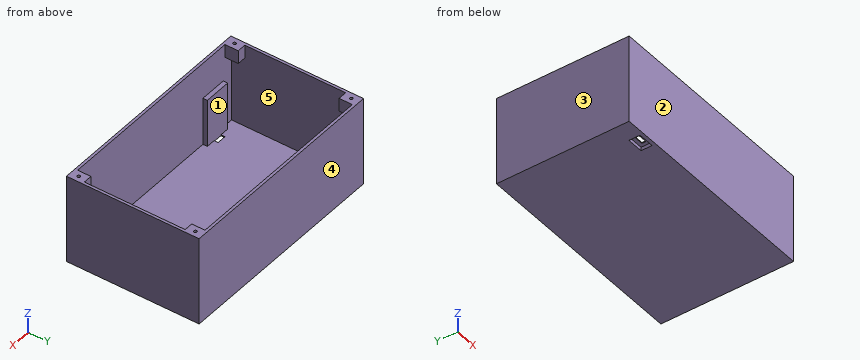
Autodesk Inventor part; units mm, degrees
ref_plane "YZ Plane" through (0, 0, 0) normal (1, 0, 0) x (0, 1, 0)
ref_plane "XZ Plane" through (0, 0, 0) normal (0, 1, 0) x (-1, 0, 0)
ref_plane "XY Plane" through (0, 0, 0) normal (0, 0, 1) x (1, 0, 0)
sketch "Sketch7" plane through (0, 0, 0) normal (0, 0, 1) x (1, 0, 0)
  line L0 (125, -75) -> (-125, -75)
  line L1 (-125, -75) -> (-125, 75)
  line L2 (-125, 75) -> (125, 75)
  line L3 (125, 75) -> (125, -75)
  line L4 (125, -75) -> (-125, 75) construction
  line L5 (-125, -75) -> (125, 75) construction
  point P0 (0, 0)
  dimension "d15" = 250
  dimension "d16" = 150
extrude "Box Outside" add sketch "Sketch7" along normal blind 100
sketch "Sketch8" plane through (0, 0, 100) normal (0, 0, 1) x (1, 0, 0)
  line L0 (-122, 72) -> (122, 72)
  line L1 (122, 72) -> (122, -72)
  line L2 (122, -72) -> (-122, -72)
  line L3 (-122, -72) -> (-122, 72)
  line L4 (125, 75) -> (-125, 75)
  line L5 (-125, 75) -> (-125, -75)
  line L6 (-125, -75) -> (125, -75)
  line L7 (125, -75) -> (125, 75)
  point P0 (0, 0)
  dimension "d19" = 3
  dimension "d20" = 3
  dimension "d21" = 3
  dimension "d22" = 3
extrude "Box Cut" cut sketch "Sketch8" against normal blind 95 contours L0 L1 L2 L3
sketch "Sketch9" plane through (-122, -72, 100) normal (0, 1, 0) x (1, 0, 0)
  line L0 (0, 0) -> (10, 0)
  line L1 (10, 0) -> (10, 15)
  line L2 (10, 15) -> (0, 15)
  line L3 (0, 15) -> (0, 0)
  point P0 (122, 100)
  dimension "d25" = 10
  dimension "d26" = 15
extrude "ScrewHole Box LB" add sketch "Sketch9" along normal blind 15
sketch "Sketch10" plane through (-122, -72, 5) normal (0, 1, 0) x (1, 0, 0)
  line L0 (244, -95) -> (244, 0)
  line L1 (244, -95) -> (234, -95)
  line L2 (234, -95) -> (234, -80)
  line L3 (234, -80) -> (244, -80)
  line L4 (244, -80) -> (244, -95)
  point P0 (122, 5)
  dimension "d29" = 10
  dimension "d30" = 15
extrude "ScrewHole Box RB" add sketch "Sketch10" along normal blind 15
sketch "Sketch11" plane through (-122, 72, 100) normal (0, -1, 0) x (1, 0, 0)
  line L0 (0, 0) -> (244, 0)
  line L1 (0, 0) -> (10, 0)
  line L2 (10, 0) -> (10, -15)
  line L3 (10, -15) -> (0, -15)
  line L4 (0, -15) -> (0, 0)
  point P0 (122, -100)
  dimension "d33" = 10
  dimension "d34" = 15
extrude "ScrewHole Box LU" add sketch "Sketch11" along normal blind 15
sketch "Sketch13" plane through (122, -72, 5) normal (-1, 0, 0) x (0, 0, 1)
  line L0 (95, 144) -> (0, 144)
  line L1 (95, 144) -> (80, 144)
  line L2 (80, 144) -> (80, 129)
  line L3 (80, 129) -> (95, 129)
  line L4 (95, 129) -> (95, 144)
  point P0 (-5, 72)
  dimension "d37" = 15
  dimension "d38" = 15
extrude "ScrewHole Box RU" add sketch "Sketch13" along normal blind 10
sketch "Sketch27" plane through (0, 0, 100) normal (0, 0, 1) x (1, 0, 0)
  line L0 (-112, -72) -> (-112, -57)
  line L1 (-125, 75) -> (-125, -75)
  line L2 (-112, -57) -> (-125, -57)
  line L3 (-125, -57) -> (-125, -75)
  line L4 (-125, -75) -> (-112, -75)
  line L5 (-112, -75) -> (-112, -57)
  line L6 (-112, -57) -> (-125, -75)
  line L7 (-112, -75) -> (-125, -57)
  circle A0 centre (-118.5, -66) radius 2.4
  point P0 (0, 0)
  dimension "d84" = 4.8
extrude "Outside ScrewHole LB" cut sketch "Sketch27" against normal blind 26 contours A0 L7 L6 | L6 L7 A0 | A0 L6 L7 | L7 L6 A0
sketch "Sketch29" plane through (0, 0, 100) normal (0, 0, 1) x (1, 0, 0)
  line L0 (-112, -72) -> (-112, -57)
  line L1 (-125, -75) -> (125, -75)
  line L2 (-112, -57) -> (-125, -57)
  line L3 (-125, -57) -> (-125, -75)
  line L4 (-125, -75) -> (-112, -75)
  line L5 (-112, -75) -> (-112, -57)
  line L6 (-112, -57) -> (-125, -75)
  circle A0 centre (-118.5, -66) radius 2.4
  point P0 (0, 0)
extrude "ScrewRibbon LB" add sketch "Sketch29" against normal blind 2 contours A0 L6 | L6 A0
sketch "Sketch30" plane through (0, 0, 100) normal (0, 0, 1) x (1, 0, 0)
  line L0 (-122, -57) -> (-112, -57)
  line L1 (-125, -75) -> (125, -75)
  line L2 (-112, -57) -> (-125, -57)
  line L3 (-125, -57) -> (-125, -75)
  line L4 (-125, -75) -> (-112, -75)
  line L5 (-112, -75) -> (-112, -57)
  line L6 (-112, -57) -> (-125, -75)
  circle A0 centre (-118.5, -66) radius 1.7
  point P0 (0, 0)
  dimension "d92" = 3.4
extrude "Inside ScrewHole LB" cut sketch "Sketch30" against normal blind 24 contours A0 L6 | L6 A0
sketch "Sketch31" plane through (0, 0, 100) normal (0, 0, 1) x (1, 0, 0)
  line L0 (-125, 75) -> (-125, -75)
  line L1 (-112, 57) -> (-122, 57)
  line L2 (-125, 75) -> (-112, 75)
  line L3 (-112, 75) -> (-112, 57)
  line L4 (-112, 57) -> (-125, 57)
  line L5 (-125, 57) -> (-125, 75)
  line L6 (-125, 75) -> (-112, 57)
  circle A0 centre (-118.5, 66) radius 2.4
  point P0 (0, 0)
  dimension "d95" = 4.8
extrude "Outside ScrewHole LU" cut sketch "Sketch31" against normal blind 24 contours A0 L6 | L6 A0
sketch "Sketch32" plane through (0, 0, 100) normal (0, 0, 1) x (1, 0, 0)
  line L0 (-122, 57) -> (-112, 57)
  line L1 (-125, 75) -> (-125, -75)
  line L2 (-112, 57) -> (-125, 57)
  line L3 (-125, 57) -> (-125, 75)
  line L4 (-125, 75) -> (-112, 75)
  line L5 (-112, 75) -> (-112, 57)
  line L6 (-112, 75) -> (-125, 57)
  circle A0 centre (-118.5, 66) radius 2.4
  point P0 (0, 0)
  dimension "d98" = 4.8
extrude "ScrewRibbon LU" add sketch "Sketch32" against normal blind 2 contours A0 L6 | L6 A0
sketch "Sketch33" plane through (0, 0, 100) normal (0, 0, 1) x (1, 0, 0)
  line L0 (125, 75) -> (-125, 75)
  line L1 (-112, 57) -> (-122, 57)
  line L2 (-125, 75) -> (-112, 75)
  line L3 (-112, 75) -> (-112, 57)
  line L4 (-112, 57) -> (-125, 57)
  line L5 (-125, 57) -> (-125, 75)
  line L6 (-125, 75) -> (-112, 57)
  circle A0 centre (-118.5, 66) radius 1.7
  point P0 (0, 0)
  dimension "d101" = 3.4
extrude "Inside ScrewHole LU" cut sketch "Sketch33" against normal blind 21.75 contours A0 L6 | L6 A0
sketch "Sketch34" plane through (0, 0, 100) normal (0, 0, 1) x (1, 0, 0)
  line L0 (112, 57) -> (112, 72)
  line L1 (125, 75) -> (-125, 75)
  line L2 (112, 57) -> (125, 57)
  line L3 (125, 57) -> (125, 75)
  line L4 (125, 75) -> (112, 75)
  line L5 (112, 75) -> (112, 57)
  line L6 (125, 75) -> (112, 57)
  circle A0 centre (118.5, 66) radius 2.4
  point P0 (0, 0)
  dimension "d104" = 4.8
extrude "Outside ScrewHole RU" cut sketch "Sketch34" against normal blind 21.75 contours A0 L6 | L6 A0
sketch "Sketch35" plane through (0, 0, 100) normal (0, 0, 1) x (1, 0, 0)
  line L0 (125, -75) -> (125, 75)
  line L1 (122, 57) -> (112, 57)
  line L2 (125, 75) -> (112, 75)
  line L3 (112, 75) -> (112, 57)
  line L4 (112, 57) -> (125, 57)
  line L5 (125, 57) -> (125, 75)
  line L6 (125, 75) -> (-125, 75)
  line L7 (125, 75) -> (112, 57)
  circle A0 centre (118.5, 66) radius 2.4
  point P0 (0, 0)
  dimension "d107" = 4.8
extrude "ScrewRibbon RU" add sketch "Sketch35" against normal blind 2 contours A0 L7 | L7 A0
sketch "Sketch36" plane through (0, 0, 100) normal (0, 0, 1) x (1, 0, 0)
  line L0 (122, 57) -> (112, 57)
  line L1 (125, -75) -> (125, 75)
  line L2 (112, 57) -> (125, 57)
  line L3 (125, 57) -> (125, 75)
  line L4 (125, 75) -> (112, 75)
  line L5 (112, 75) -> (112, 57)
  line L6 (112, 57) -> (125, 75)
  circle A0 centre (118.5, 66) radius 2.4
  circle A1 centre (118.5, 66) radius 1.7
  point P0 (0, 0)
  dimension "d110" = 3.4
extrude "Inside ScrewHole RU" cut sketch "Sketch36" against normal blind 20 contours A1 L6 | L6 A1
sketch "Sketch37" plane through (0, 0, 100) normal (0, 0, 1) x (1, 0, 0)
  line L0 (125, -75) -> (125, 75)
  line L1 (112, -72) -> (112, -57)
  line L2 (125, -75) -> (112, -75)
  line L3 (112, -75) -> (112, -57)
  line L4 (112, -57) -> (125, -57)
  line L5 (125, -57) -> (125, -75)
  line L6 (112, -75) -> (125, -57)
  circle A0 centre (118.5, -66) radius 2.4
  point P0 (0, 0)
  dimension "d113" = 4.8
extrude "Outside ScrewHole RB" cut sketch "Sketch37" against normal blind 20 contours A0 L6 | L6 A0
sketch "Sketch38" plane through (0, 0, 100) normal (0, 0, 1) x (1, 0, 0)
  line L0 (122, -57) -> (112, -57)
  line L1 (125, -75) -> (125, 75)
  line L2 (112, -57) -> (125, -57)
  line L3 (125, -57) -> (125, -75)
  line L4 (125, -75) -> (112, -75)
  line L5 (112, -75) -> (112, -57)
  line L6 (125, -57) -> (112, -75)
  circle A0 centre (118.5, -66) radius 2.4
  point P0 (0, 0)
  dimension "d116" = 4.8
extrude "ScrewRibbon RB" add sketch "Sketch38" against normal blind 2 contours A0 L6 | L6 A0
sketch "Sketch39" plane through (0, 0, 100) normal (0, 0, 1) x (1, 0, 0)
  line L0 (112, -72) -> (112, -57)
  line L1 (125, -75) -> (125, 75)
  line L2 (112, -57) -> (125, -57)
  line L3 (125, -57) -> (125, -75)
  line L4 (125, -75) -> (112, -75)
  line L5 (112, -75) -> (112, -57)
  line L6 (112, -75) -> (125, -57)
  circle A0 centre (118.5, -66) radius 2.4
  circle A1 centre (118.5, -66) radius 1.7
  point P0 (0, 0)
  dimension "d119" = 3.4
extrude "Inside ScrewHole RB" cut sketch "Sketch39" against normal blind 20 contours A1 L6 | L6 A1
sketch "Sketch42" plane through (-122, -72, 5) normal (0, 1, 0) x (1, 0, 0)
  line L0 (244, 0) -> (0, 0)
  line L1 (12.5963, 0) -> (43.5963, 0)
  line L2 (43.5963, 0) -> (43.5963, -54)
  line L3 (43.5963, -54) -> (12.5963, -54)
  line L4 (12.5963, -54) -> (12.5963, 0)
  point P0 (122, 5)
  point P1 (43.5963, 0)
  dimension "d134" = 31
  dimension "d135" = 54
extrude "ESPHolder" add sketch "Sketch42" along normal blind 5
sketch "Sketch43" plane through (0, 0, 5) normal (0, 0, 1) x (1, 0, 0)
  line L0 (-109.4037, -67) -> (-78.4037, -67)
  line L1 (-99.1037, -67) -> (-88.7037, -67)
  line L2 (-88.7037, -67) -> (-88.7037, -62.5)
  line L3 (-88.7037, -62.5) -> (-99.1037, -62.5)
  line L4 (-99.1037, -62.5) -> (-99.1037, -67)
  line L5 (-78.4037, -67) -> (-109.4037, -67)
  line L6 (-109.4037, -67) -> (-109.4037, -51.7804)
  line L7 (-109.4037, -51.7804) -> (-78.4037, -51.7804)
  line L8 (-78.4037, -51.7804) -> (-78.4037, -67)
  point P0 (0, 0)
  dimension "d138" = 10.3
  dimension "d139" = 10.3
  dimension "d140" = 4.5
extrude "PortHole" cut sketch "Sketch43" against normal through all contours L4 L3 L2 L0
sketch "Sketch44" plane through (0, 0, 0) normal (0, 0, -1) x (-1, 0, 0)
  line L0 (84.7037, -58.5) -> (103.1037, -58.5)
  line L1 (103.1037, -58.5) -> (103.1037, -71)
  line L2 (103.1037, -71) -> (84.7037, -71)
  line L3 (84.7037, -71) -> (84.7037, -58.5)
  line L4 (88.7037, -62.5) -> (99.1037, -62.5)
  line L5 (99.1037, -67) -> (88.7037, -67)
  line L6 (99.1037, -62.5) -> (99.1037, -67)
  line L7 (88.7037, -67) -> (88.7037, -62.5)
  point P0 (0, 0)
  dimension "d143" = 4
  dimension "d144" = 4
  dimension "d145" = 4
  dimension "d146" = 4
extrude "Extrusion29" cut sketch "Sketch44" against normal blind 4
properties part number "Box"
Could you check a few things on this model? Use its own coordinates, in mm. Face numbers are marked on the shaded views. A direction names the side the tool comes from. Coordinates: 2 decimals unless noted, no trailing zeros. Order: outer loops, then holes, each group sorted by start corner. A loop starts at its lowest first (then second) coordinate and runs counter-clockwise, first axis right, second up. Notation, with made-up numbers: (65, 58) -> (114, 58) arc R17 ccw to (114, 72) -> close; hole circle Ø2 at (40.5, 66.5). An arc over 180 degrees is marked (long way). One line per item, written item: value. Start each with the question number.
1) Which directions (+Z, -Z, +X, -X, +Y, -Y) give clear straight access to the entire face, cutting with the end or side of a thin tool? Please do the marked faces 4 and 5.
2) Imagine slicing it at C-C on y = 38. List the corners of the cut face in (x, z) for me, plus the area to 3 significant figures.
3) If I drill on L1, parallel to X at y = -66, z = 98.5; L2, parallel to Y at x = 118.5, z = 93.5; L3, parallel to Y at x = 118.5, z = 98.6, over which ranges is the centre line in solid material (lowest first)? Write a range as [from, to].
4) I'm going to push flat-ended pins straight in: pin 1 (2 mm diameter, centred on x = 118.5, y = -66, fed in from +Z); pin 2 (11 mm diameter, centred on x = 119.5, y = -62, fed in from -Z). Where does each tip first touch, or does it pass through?
5) We'd pull the mould along X, two halves only. Please class the marked faces 1, 2 and 3: +X half, -X half, draft (parallel to the pull), parting line (faces both ways), or undercut.
6) Imagine slicing it at B-B on x = 94.5. List the corners of the cut face in (y, z) for me.
7) Imagine slicing it at A-A on z = 37.5. List the corners of the cut face in (x, y) for me.
Answer list:
1. face 4: +Z, -Z, +X, -X, +Y
1. face 5: none
2. outline: (-125, 0) -> (125, 0) -> (125, 100) -> (122, 100) -> (122, 5) -> (-122, 5) -> (-122, 100) -> (-125, 100) -> close
2. area: 1,820 mm2
3. L1: x = [-125, -120.2], [-116.8, -112], [112, 116.8], [120.2, 125]
3. L2: y = [-75, -68.4], [-63.6, -57], [57, 63.6], [68.4, 75]
3. L3: y = [-75, -67.7], [-64.3, -57], [57, 64.3], [67.7, 75]
4. pin 1: stops at z = 5
4. pin 2: stops at z = 0
5. face 1: undercut
5. face 2: draft
5. face 3: -X half
6. outline: (-75, 0) -> (75, 0) -> (75, 100) -> (72, 100) -> (72, 5) -> (-72, 5) -> (-72, 100) -> (-75, 100) -> close
7. outline: (-125, -75) -> (125, -75) -> (125, 75) -> (-125, 75) -> close; hole (-122, -72) -> (-109.4, -72) -> (-109.4, -67) -> (-78.4, -67) -> (-78.4, -72) -> (122, -72) -> (122, 72) -> (-122, 72) -> close
